from build123d import *

# Parameters (mm, degrees)
BOSS_EXTRUDE1_DEPTH     = 2
CUT_EXTRUDE1_DEPTH      = 22.271988328
CUT_EXTRUDE1_DEPTH_BACK = 22.271988328


with BuildPart() as part:
    # Sketch1 → Boss-Extrude1 (new body)
    with BuildSketch(Plane(origin=(0, 0, 0), x_dir=(1, 0, 0), z_dir=(0, 1, 0))):
        with BuildLine():
            Line((-0.5, 4.974937186), (-0.5, 14.974937186))
            Line((-0.5, 14.974937186), (0.5, 14.974937186))
            Line((0.5, 14.974937186), (0.5, 4.974937186))
            ThreePointArc((0.5, 4.974937186), (3.535533906, 3.535533906), (4.974937186, 0.5))
            Line((4.974937186, 0.5), (14.974937186, 0.5))
            Line((14.974937186, 0.5), (14.974937186, -0.5))
            Line((14.974937186, -0.5), (4.974937186, -0.5))
            ThreePointArc((4.974937186, -0.5), (3.535533906, -3.535533906), (0.5, -4.974937186))
            Line((0.5, -4.974937186), (0.5, -14.974937186))
            Line((0.5, -14.974937186), (-0.5, -14.974937186))
            Line((-0.5, -14.974937186), (-0.5, -4.974937186))
            ThreePointArc((-0.5, -4.974937186), (-3.535533906, -3.535533906), (-4.974937186, -0.5))
            Line((-4.974937186, -0.5), (-14.974937186, -0.5))
            Line((-14.974937186, -0.5), (-14.974937186, 0.5))
            Line((-14.974937186, 0.5), (-4.974937186, 0.5))
            ThreePointArc((-4.974937186, 0.5), (-3.535533906, 3.535533906), (-0.5, 4.974937186))
        make_face()
    extrude(amount=BOSS_EXTRUDE1_DEPTH)

    # Sketch2 → Cut-Extrude1 (cut, two sides: drawn at the far end of the back side and taken through both)
    with BuildSketch(Plane(origin=(0, 0, 0), x_dir=(1, 0, 0), z_dir=(0, 1, 0)).offset(-CUT_EXTRUDE1_DEPTH_BACK)):
        with BuildLine():
            Line((-3, -2.645751311), (-3, 2.645751311))
            ThreePointArc((-3, 2.645751311), (4, 0), (-3, -2.645751311))
        make_face()
    extrude(amount=CUT_EXTRUDE1_DEPTH + CUT_EXTRUDE1_DEPTH_BACK, mode=Mode.SUBTRACT)


solid = part.part
The model under review builds one solid part; all positions refer to its coordinate system, in mm. A direction names the side the tool comes from. Give positions to 0.01 mm unless a question says otherwise; leave off trailing zeros. Write each loop counter-clockwise with the first axis right and the second up, starting at its lowest first coordinate (ties: lowest second). Pieces come first, ordered by that corner, then holes. Notation, with made-up numbers: M -31,57 L 6,57 A27 cw 6,75 Z; hole C -5,82 d5. An arc over 180 degrees is marked long. One line per question, with ' | ' between items. Start each with the question number.
Item 1: We need section A-A on y = 0.8. Write out the cut boundary in (x, z), plus the area to 3 significant figures.
Item 2: We need section B-B on z = 0. Write out the cut boundary in (x, y), plus the area to 3 significant figures.
Item 3: Draft analysis for pull direction X (two halves, no side actions). For faces 1 (the cylindrical face through (4, 1, 0)), 2 (the flat face through (-3, 1, 0)), 3 (the flat face through (-3.3, 2, -0.1)), 4 (the flat face through (0.5, 1, 10)), state which applies: released by +X, released by -X, zero draft, split by the parting line, or undercut.
Item 4: Wall thickness on line 1 (Z direction, x = 0, y = 0.45); line 2 (X direction, y = 0.4, z = 0); line 3 (Z direction, x = -2, y = 1.05): over which ranges is each line inside the solid? List them lowest first. Write a range as from..to.
Item 5: We need section C-C on x = 0. Write out the cut boundary in (y, z).
Item 6: We need section D-D on x = -11.25. Write out the cut boundary in (y, z).
Item 7: For pin 1 (0.6 mm diameter, centred on x = 9.5, y = 0.5, fed in from +Z); pin 2 (1 mm diameter, centred on x = -7.5, y = 0.5, fed in from -Z); pin 3 (1 mm diameter, centred on y = 0.5, z = 7.5, fed in from -X), all flat-tipped, find the tip position at first contact; note any pin that passes through.
Item 8: For faces 5 (the flat face through (0.5, 1, -10)), 6 (the flat face through (-10, 1, -0.5)), 7 (the flat face through (-10, 1, 0.5)), list the 3-axis set-ups (+Z, -Z, +X, -X, +Y, -Y) from which the entire face can be reached by the end or side of a thin tool; tool diameter is ignored.
Results found:
1) outline: M -14.97,-0.5 L -4.97,-0.5 A5 ccw -0.5,-4.97 L -0.5,-14.97 L 0.5,-14.97 L 0.5,-4.97 A5 ccw 4.97,-0.5 L 14.97,-0.5 L 14.97,0.5 L 4.97,0.5 A5 ccw 0.5,4.97 L 0.5,14.97 L -0.5,14.97 L -0.5,4.97 A5 ccw -4.97,0.5 L -14.97,0.5 Z; hole M -3,-2.65 A4 ccw long -3,2.65 Z | area: 71.8 mm2
2) outline: M -14.97,0 L -3,0 L -3,2 L -14.97,2 Z; M 4,0 L 14.97,0 L 14.97,2 L 4,2 Z | area: 45.9 mm2
3) face 1: undercut | face 2: undercut | face 3: zero draft | face 4: released by +X
4) line 1: z = -14.97..-4, 4..14.97 | line 2: x = -14.97..-3, 4..14.97 | line 3: z = -4.58..-3.46, 3.46..4.58
5) outline: M 0,-14.97 L 2,-14.97 L 2,-4 L 0,-4 Z; M 0,4 L 2,4 L 2,14.97 L 0,14.97 Z
6) outline: M 0,-0.5 L 2,-0.5 L 2,0.5 L 0,0.5 Z
7) pin 1: stops at z = 0.5 | pin 2: stops at z = -0.5 | pin 3: stops at x = -0.5
8) face 5: -Z, +X, +Y, -Y | face 6: -Z, -X, +Y, -Y | face 7: +Z, -X, +Y, -Y
